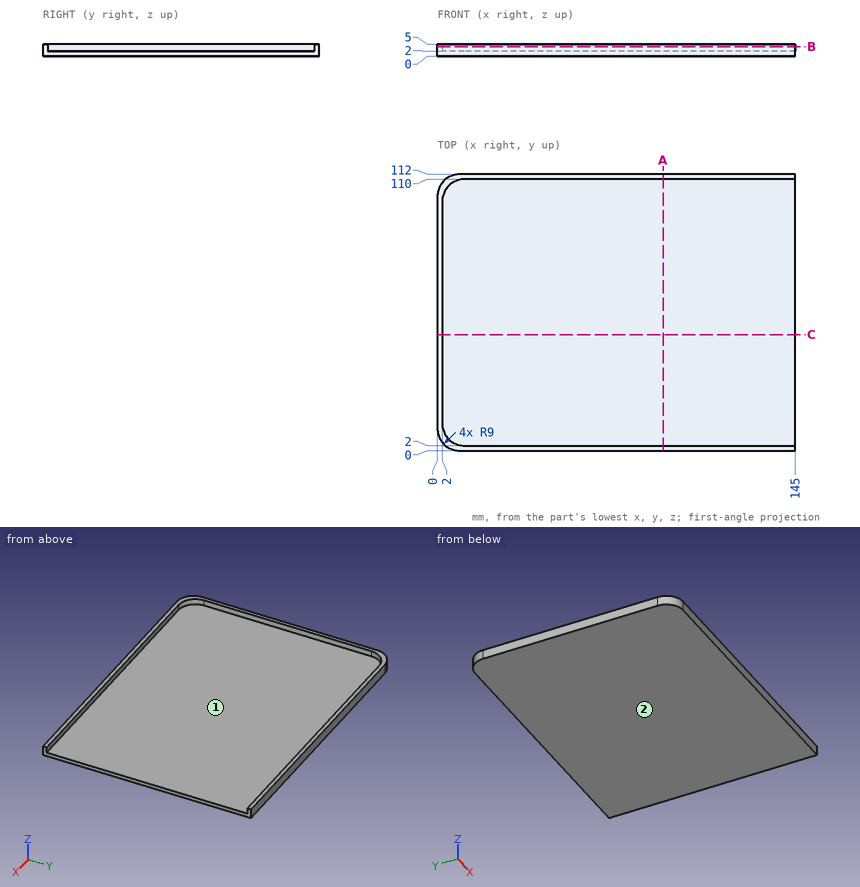
Geometry: see drawing. Coordinates: mm, zero at the bounding-box minimum. Round coordinates to 2 decimals unless told otherwise and drop trailing zeros. Write each loop counter-clockwise with the first axis right and the second up, starting at its lowest first coordinate (ties: lowest second). Pieces come first, ordered by that corner, then holes.
1) Draft query along Y for the marked faces 1 and 2. Return one class per face: pulls with the +Y half, pulls with the -Y half, needs draft (parallel to the pull), parting line crosses it, or undercut.
2) Ray query, L1, parallel to Y at x = 94.5, z = 2.3; L2, parallel to Z at x = 93, y = 82. Return the intervals inside material, ascending.
3) Cut plane A-A (x = 91.5). Return the cut outline in (y, z), then the cut area to 3 significant figures.
4) Cut plane B-B (z = 3.9). Return the cut outline in (x, y), then the cut area to 3 significant figures.
5) Contact query for flat-ended pins moving along their axis: P1, Ø2.5, axis at y = 77, z = 3.5, coming from the +X side; P2, Ø3, axis at x = 65, y = 32, coming from the +Z side. Output: stop coordinate, or through.
6) Cut plane C-C (y = 47). Return the cut outline in (x, z).
Geometry says:
1. face 1: undercut
1. face 2: needs draft
2. L1: y = 0 to 2, 110 to 112
2. L2: z = 0 to 2
3. outline: (0, 0) - (112, 0) - (112, 5) - (110, 5) - (110, 2) - (2, 2) - (2, 5) - (0, 5) - close
3. area: 236 mm2
4. outline: (0, 9) arc R9 ccw to (9, 0) - (145, 0) - (145, 2) - (11, 2) arc R9 cw to (2, 11) - (2, 101) arc R9 cw to (11, 110) - (145, 110) - (145, 112) - (9, 112) arc R9 ccw to (0, 103) - close
4. area: 796 mm2
5. P1: stops at x = 2
5. P2: stops at z = 2
6. outline: (0, 0) - (145, 0) - (145, 2) - (2, 2) - (2, 5) - (0, 5) - close
